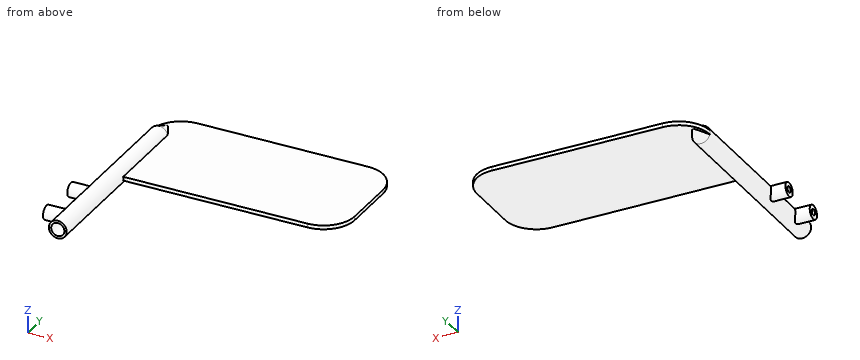
Autodesk Inventor part; units mm, degrees
ref_plane "YZ Plane" through (0, 0, 0) normal (1, 0, 0) x (0, 1, 0)
ref_plane "XZ Plane" through (0, 0, 0) normal (0, 1, 0) x (-1, 0, 0)
ref_plane "XY Plane" through (0, 0, 0) normal (0, 0, 1) x (1, 0, 0)
sketch "Skizze1" plane through (0, 0, 0) normal (0, 1, 0) x (-1, 0, 0)
  circle A0 centre (0, 0) radius 8.5
  circle A1 centre (0, 0) radius 11.5
  dimension "d0" = 17
  dimension "d1" = 3
extrude "Extrusion1" add sketch "Skizze1" along normal blind 250
sketch "Skizze2" plane through (0, 0, 0) normal (0, 0, 1) x (1, 0, 0)
  line L0 (11.5, 250) -> (-11.5, 250)
  line L1 (-11.5, 250) -> (-11.5, 250)
  line L2 (28.5, 290) -> (248.5, 290)
  line L3 (288.5, 250) -> (288.5, 180)
  line L4 (248.5, 140) -> (8.5, 140)
  line L5 (8.5, 250) -> (8.5, 0)
  arc A0 (248.5, 140) -> (288.5, 180) centre (248.5, 180) ccw
  arc A1 (288.5, 250) -> (248.5, 290) centre (248.5, 250) ccw
  arc A2 (28.5, 290) -> (-11.5, 250) centre (28.5, 250) ccw
  point P0 (0, 0)
  point P1 (-11.5, 290)
  point P2 (288.5, 290)
  point P3 (288.5, 140)
  dimension "d4" = 40
  dimension "d5" = 300
  dimension "d6" = 150
  dimension "d7" = 40
extrude "Extrusion2" add sketch "Skizze2" along normal mid plane 5
sketch "Skizze3" plane through (0, 0, 0) normal (1, 0, 0) x (0, 1, 0)
  line L0 (250, -11.5) -> (250, -2.5)
  line L1 (250, -2.5) -> (180, -2.5)
  line L2 (250, -2.5) -> (250, -2.5)
  line L3 (250, -2.5) -> (250, -11.5)
  line L4 (-70, 0) -> (420, 0)
  line L5 (250, -11.5) -> (270, -2.5)
  line L6 (250, -2.5) -> (290, -2.5)
  point P0 (0, 0)
revolve "Umdrehung1" add sketch "Skizze3" angle 360 about axis through (0, -10, 0) along (0, 1, 0)
sketch "Skizze4" plane through (0, 0, 0) normal (1, 0, 0) x (0, 1, 0)
  line L0 (0, 0) -> (30, 0)
  line L1 (30, 0) -> (90, 0)
  circle A0 centre (30, 0) radius 5
  circle A1 centre (90, 0) radius 5
  dimension "d11" = 30
  dimension "d12" = 60
  dimension "d13" = 10
  dimension "d14" = 10
extrude "Extrusion3" cut sketch "Skizze4" against normal through all
sketch "Skizze5" plane through (0, 0, 0) normal (1, 0, 0) x (0, 1, 0)
  line L0 (0, 0) -> (30, 0)
  circle A0 centre (30, 0) radius 4
  circle A1 centre (30, 0) radius 9
  line L1 (30, 0) -> (90, 0)
  circle A2 centre (90, 0) radius 4
  circle A3 centre (90, 0) radius 9
  dimension "d17" = 30
  dimension "d18" = 8
  dimension "d19" = 5
  dimension "d20" = 60
  dimension "d21" = 8
  dimension "d22" = 5
extrude "Extrusion4" add sketch "Skizze5" against normal blind 30 contours A1 L1 A0 L0 | A3 | L0 A0 L1 A1
sketch "Skizze6" plane through (0, 0, 0) normal (0, -1, 0) x (1, 0, 0)
  circle A0 centre (0, 0) radius 8.5
  dimension "d25" = 17
extrude "Extrusion5" cut sketch "Skizze6" against normal blind 250
thread "Gewinde3"
thread "Gewinde4"
properties part number "HTW-000692" material "PVC, hart"
Design review of the part built by this model. Coordinates are the model's own, in mm. Coordinates: 2 decimals unless noted, no trailing zeros. Order: outer loops, then holes, each group sorted by start corner. A loop starts at its lowest first (then second) coordinate and runs counter-clockwise, first axis right, second up. Notation, with made-up numbers: M 59,5.25 L 80,5.25 A10 ccw 80,15.25 Z; hole C 25,19.25 d11. An arc over 180 degrees is marked long. Answer as a JSON object with one key per item and string values. Group by question number.
1) For pin 1 (4 mm diameter, centred on y = 148, z = -3, fed in from -X); pin 2 (1.5 mm diameter, centred on x = 100, z = 3, fed in from -Y); pin 3 (1 mm diameter, centred on x = 63, y = 234.5, fed in from -Z); pin 4 (13 mm diameter, centred on y = 30, z = 0, fed in from -X), all flat-tipped, find the tip position at first contact; note any pin that passes through.
2) Add section B-B, the plane x = 143.5. Write out the cut boundary in (y, z), then the cut area to 3 significant figures.
3) Wall thickness on L1, parallel to Y at x = -23, z = 0; L2, parallel to Z at x = 0, y = 190; L3, parallel to Z at x = -13.25, y = 90: over which ranges is each line inside the solid? List them lowest first.
4) Add section D-D, the plane y = 45.5. Write out the cut boundary in (x, z).
5) Add section C-C, the plane y = 161. Write out the cut boundary in (x, z), then the cut area to 3 significant figures.
6) Add section A-A, the plane y = 203. Write out the cut boundary in (x, z), then the cut area to 3 significant figures.
Computed values:
{
 "1": {"pin 1": "stops at x = -11.46", "pin 2": "stops at y = 140", "pin 3": "stops at z = -2.5", "pin 4": "stops at x = -30"},
 "2": {"outline": "M 140,-2.5 L 290,-2.5 L 290,2.5 L 140,2.5 Z", "area": "750 mm^2"},
 "3": {"L1": "y = 21 to 26, 34 to 39, 81 to 86, 94 to 99", "L2": "z = -11.5 to -8.5, 8.5 to 11.5", "L3": "z = -9 to -4, 4 to 9"},
 "4": {"outline": "C 0,0 d23; hole C 0,0 d17"},
 "5": {"outline": "M 11.22,-2.5 L 283.7,-2.5 L 283.7,2.5 L 11.22,2.5 A11.5 ccw long Z; hole C 0,0 d17", "area": "1,550 mm^2"},
 "6": {"outline": "M 11.22,-2.5 L 288.5,-2.5 L 288.5,2.5 L 11.22,2.5 A11.5 ccw long Z; hole C 0,0 d17", "area": "1,570 mm^2"}
}
